Verification items for the finished model (mm, model axes). Face numbers are marked on the shaded views. A direction names the side the tool comes from. Round coordinates to 2 decimals unless told otherwise and drop trailing zeros. Loops run counter-clockwise (first coordinate to the right, second up) from the corner with the lowest first, then second, coordinate; pieces in that order, holes last. Notation, with made-up numbers: M 24,48 L 38,48 A17 cw 38,80 Z; hole C 51,1 d2. An arc over 180 degrees is marked long. Write item = value, one per line. Start each with the question number.
Autodesk Inventor part; units mm, degrees
ref_plane "YZ Plane" through (0, 0, 0) normal (1, 0, 0) x (0, 1, 0)
ref_plane "XZ Plane" through (0, 0, 0) normal (0, 1, 0) x (-1, 0, 0)
ref_plane "XY Plane" through (0, 0, 0) normal (0, 0, 1) x (1, 0, 0)
sketch "Sketch2" plane through (0, 0, 0) normal (0, 1, 0) x (-1, 0, 0)
  line L0 (0, 0) -> (-25.4, 0)
  line L1 (-25.4, 0) -> (-25.4, -50.8)
  line L2 (-25.4, -50.8) -> (0, -50.8)
  line L3 (0, -50.8) -> (0, 0)
  line L4 (-1.778, -1.778) -> (-23.622, -1.778)
  line L5 (-23.622, -1.778) -> (-23.622, -49.022)
  line L6 (-23.622, -49.022) -> (-1.778, -49.022)
  line L7 (-1.778, -49.022) -> (-1.778, -1.778)
  dimension "d0" = 25.4
  dimension "d1" = 50.8
  dimension "d2" = 1.778
extrude "Extrusion1" add sketch "Sketch2" along normal blind 93.345
sketch "Sketch3" plane through (25.4, 0, 0) normal (1, 0, 0) x (0, 0, -1)
  line L0 (1.778, 0) -> (49.022, 0) construction
  line L1 (25.4, 0) -> (25.4, 48.768) construction
  line L2 (25.4, 48.768) -> (25.4, 74.168) construction
  circle A0 centre (25.4, 74.168) radius 14.2875
  point P0 (0, 0)
  dimension "d5" = 48.768
  dimension "d6" = 25.4
  dimension "d7" = 28.575
extrude "Extrusion2" cut sketch "Sketch3" against normal blind 42.545
sketch "Sketch4" plane through (25.4, 0, 0) normal (1, 0, 0) x (0, 0, -1)
  line L0 (0, 0) -> (12.7, 0) construction
  line L1 (50.8, 0) -> (0, 0) construction
  line L2 (12.7, 0) -> (25.4, 0) construction
  line L3 (25.4, 0) -> (38.1, 0) construction
  line L4 (12.7, 0) -> (12.7, 12.7) construction
  line L5 (12.7, 12.7) -> (12.7, 25.4) construction
  circle A0 centre (12.7, 25.4) radius 2.5797
  circle A1 centre (12.7, 12.7) radius 2.5797
  line L6 (12.7, 25.4) -> (25.4, 25.4) construction
  line L7 (25.4, 25.4) -> (38.1, 25.4) construction
  line L8 (25.4, 12.7) -> (25.4, 25.4) construction
  circle A2 centre (25.4, 25.4) radius 2.5797
  circle A3 centre (25.4, 12.7) radius 2.5797
  line L9 (38.1, 12.7) -> (38.1, 25.4) construction
  circle A4 centre (38.1, 25.4) radius 2.5797
  circle A5 centre (38.1, 12.7) radius 2.5797
  dimension "d10" = 12.7
  dimension "d11" = 12.7
  dimension "d12" = 12.7
  dimension "d13" = 12.7
  dimension "d14" = 12.7
  dimension "d15" = 5.1594
  dimension "d16" = 5.1594
  dimension "d17" = 12.7
  dimension "d27" = 12.7
  dimension "d28" = 12.7
  dimension "d29" = 5.1594
  dimension "d30" = 5.1594
  dimension "d31" = 12.7
  dimension "d32" = 5.1594
  dimension "d33" = 5.1594
extrude "Extrusion3" cut sketch "Sketch4" against normal blind 25.4
properties part number "anchor point"
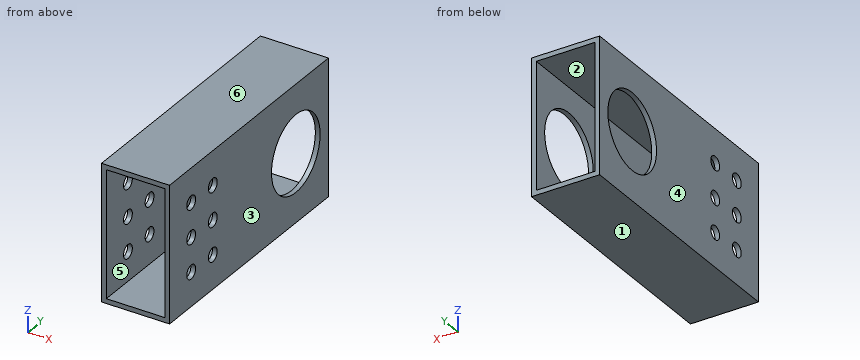
1. Section check A-A, the plane z = -45. Enter the section's corners in (x, y) (3 decimals).
2. Section check B-B, the plane x = 22.5. Enter the section's corners in (y, z) (3 decimals), and give its area (3 significant figures).
3. Gauge pin test, flat end, axial feed: P1, Ø3, axis at y = 25.4, z = -38.1, coming from the -X side. Record the tip position at first contact, or that the pin passes through.
4. Thickness scan on line 1 (Y direction, x = 25, z = -25.4) (1 decimal); line 2 (X direction, y = 17, z = -47); line 3 (Z direction, x = 23.5, y = 44.5). Record the ranges inside material, lowest first.
5. Tool access check on the marked faces 5 and 6. Record the directions out of +Z, -Z, +X, -X, +Y, -Y that give a thin tool (end or side, any length) a straight path to the whole face; none if there is none.
6. Mould release check, pull along X, two halves, no side actions. Record for the marked faces 1, 2, 3 and 4: pulls with the +X half, pulls with the -X half, needs draft (parallel to the pull), parting line crosses it, or undercut.
7. Section check C-C, the plane z = -25.4. Give the number of separate pieces and of enclosed holes in the cut face, and give its area (3 significant figures).
Computed values:
q1.outline = M 0,0 L 1.778,0 L 1.778,93.345 L 0,93.345 Z; M 23.622,0 L 25.4,0 L 25.4,93.345 L 23.622,93.345 Z
q2.outline = M 0,-50.8 L 93.345,-50.8 L 93.345,-49.022 L 0,-49.022 Z; M 0,-1.778 L 93.345,-1.778 L 93.345,0 L 0,0 Z
q2.area = 332 mm2
q3.P1 = through
q4.line_1 = 0 to 10.1, 15.3 to 22.8, 28 to 59.9, 88.5 to 93.3
q4.line_2 = 0 to 1.78, 23.62 to 25.4
q4.line_3 = -50.8 to -49.02, -1.78 to 0
q5.face_5 = +Y, -Y
q5.face_6 = +Z, +X, -X, +Y, -Y
q6.face_1 = needs draft
q6.face_2 = undercut
q6.face_3 = pulls with the +X half
q6.face_4 = pulls with the -X half
q7.separate_pieces = 8
q7.enclosed_holes = 0
q7.area = 194 mm2
